Input: dimensioned drawing with shaded views. Units: mm. Origin: part minimum x, y, z. Coordinates: 2 decimals unless noted, no trailing zeros. Write each loop counter-clockwise with the first axis right and the second up, starting at its lowest first coordinate (ties: lowest second). Pieces come first, ordered by that corner, then holes. Notation, with made-up numbers: (48, 3) -> (61, 3) arc R31 cw to (61, 40) -> close; hole circle Ø10 at (-6.5, 40). An arc over 180 degrees is marked (long way). One line per item, written item: value. Start each with the question number.
1. Section query B-B, the plane x = 130.5. Output: boundary loops of the cut face in (y, z) (1 decimal).
2. Section query C-C, the plane x = 17.5. Output: boundary loops of the cut face in (y, z).
3. First-contact query: P1, Ø0.9, axis at y = 3, z = 110.5, coming from the -X side; P2, Ø4, axis at x = 33.5, z = 157, coming from the +Y side; P3, Ø1.5, axis at y = 4, z = 84, coming from the +X side (1 decimal). Flat tips, straight axial feed; report the tip coordinate or a pass-through.
4. Mould query, pull axis X, two halves, no side actions, for the marked faces 1 and 2. Classes: released by +X, released by -X, zero draft, split by the parting line, or undercut.
5. Section query A-A, the plane y = 33. Output: boundary loops of the cut face in (x, z) (1 decimal), and give its area (3 significant figures).
6. Line query: line 1 (X direction, y = 28, z = 100.5) (1 decimal); line 2 (Y direction, x = 112, z = 55); line 3 (Y direction, x = 121.5, z = 192). Output: solid intervals per line, ascending.
7. Section query D-D, the plane y = 7.5. Output: boundary loops of the cut face in (x, z) (1 decimal).
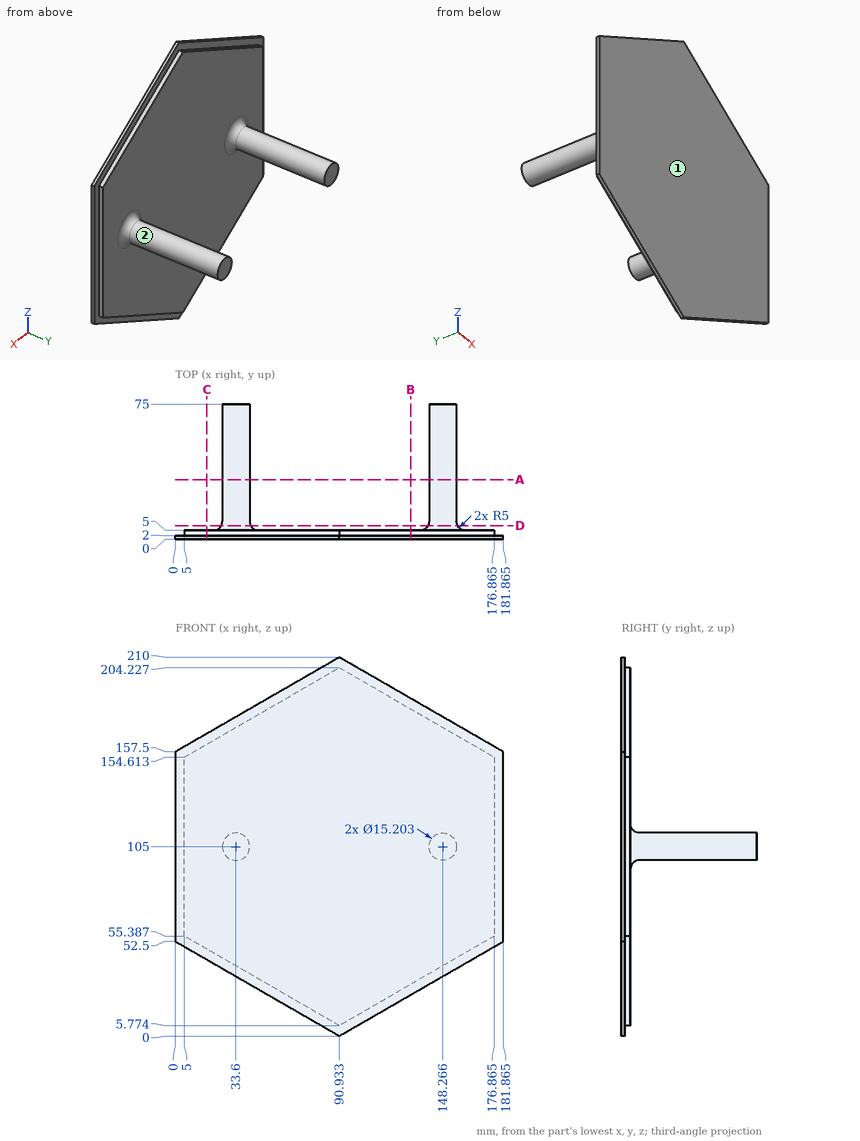
Computed values:
1. outline: (0, 22.8) -> (2, 22.8) -> (2, 28.6) -> (5, 28.6) -> (5, 181.4) -> (2, 181.4) -> (2, 187.2) -> (0, 187.2) -> close
2. outline: (0, 42.4) -> (2, 42.4) -> (2, 48.17) -> (5, 48.17) -> (5, 161.83) -> (2, 161.83) -> (2, 167.6) -> (0, 167.6) -> close
3. P1: stops at x = 5
3. P2: stops at y = 5
3. P3: stops at x = 176.9
4. face 1: zero draft
4. face 2: undercut
5. outline: circle Ø15.2 at (33.6, 105); circle Ø15.2 at (148.3, 105)
5. area: 363 mm²
6. line 1: x = 27.5 to 39.7, 142.1 to 154.4
6. line 2: y = 0 to 5
6. line 3: y = 0 to 2
7. outline: circle Ø16.5 at (33.6, 105); circle Ø16.5 at (148.3, 105)
